```python
from build123d import *

# Parameters (mm, degrees)
F0_W      = 15.2
F0_H      = 19.2
F1_DEPTH  = 1.6
F2_R      = 1
F3_DEPTH  = 25
F4_W      = 10
F4_H      = 2.5
F5_DEPTH  = 2.5
F7_W      = 0.6
F7_H      = 0.6
F8_DEPTH  = 7.3
F9_W      = 0.6
F9_H      = 0.6
F10_DEPTH = 7.5
F11_R     = 3.473111
F12_DEPTH = 1
F13_R     = 2.5
F14_DEPTH = 7.5
F15_R     = 2.5


with BuildPart() as f1:
    # F0 (on Top) → F1 (new body)
    with BuildSketch(Plane.XY):
        Rectangle(F0_W, F0_H)
    extrude(amount=F1_DEPTH)

    # F2 (on face) → F3 (cut)
    with BuildSketch(Plane.XY.offset(1.6)):
        with Locations((-5.1, 7.1)):
            Circle(F2_R)
        with Locations((5.1, 7.1)):
            Circle(F2_R)
    extrude(amount=-F3_DEPTH, mode=Mode.SUBTRACT)

    # F4 (on face) → F5 (join)
    with BuildSketch(Plane.XY.offset(1.6)):
        with Locations((0, -7.85)):
            Rectangle(F4_W, F4_H)
    extrude(amount=F5_DEPTH)

    # F7 (on offset) → F8 (join)
    with BuildSketch(Plane.XY.offset(-1.5)):
        with Locations((3.85, -7.85)):
            Rectangle(F7_W, F7_H)
        with Locations((-3.85, -7.85)):
            Rectangle(F7_W, F7_H)
        with Locations((-1.35, -7.85)):
            Rectangle(F7_W, F7_H)
        with Locations((1.35, -7.85)):
            Rectangle(F7_W, F7_H)
        with Locations((1.35, -1.45)):
            Rectangle(F7_W, F7_H)
        with Locations((-1.35, -1.45)):
            Rectangle(F7_W, F7_H)
        with Locations((0, 1.45)):
            Rectangle(F7_W, F7_H)
        with Locations((-2.7, 1.45)):
            Rectangle(F7_W, F7_H)
    extrude(amount=F8_DEPTH)

    # F9 (on face) → F10 (join)
    with BuildSketch(Plane(origin=(0, -7.55, 0), x_dir=(-1, 0, 0), z_dir=(0, 1, 0))):
        with Locations((3.85, 5.5)):
            Rectangle(F9_W, F9_H)
        with Locations((-3.85, 5.5)):
            Rectangle(F9_W, F9_H)
        with Locations((1.35, 5.5)):
            Rectangle(F9_W, F9_H)
        with Locations((-1.35, 5.5)):
            Rectangle(F9_W, F9_H)
    extrude(amount=-F10_DEPTH)

    # F11 (on face) → F12 (join)
    with BuildSketch(Plane.XY.offset(5.8)):
        Circle(F11_R)
    extrude(amount=F12_DEPTH)

    # F13 (on face) → F14 (join)
    with BuildSketch(Plane.XY.offset(6.8)):
        Circle(F13_R)
    extrude(amount=F14_DEPTH)

    # F15
    f15_edges = [f1.edges().sort_by_distance(p)[0] for p in [
        (-2.5, 0, 14.3),
    ]]
    fillet(f15_edges, radius=F15_R)


solid = f1.part
```
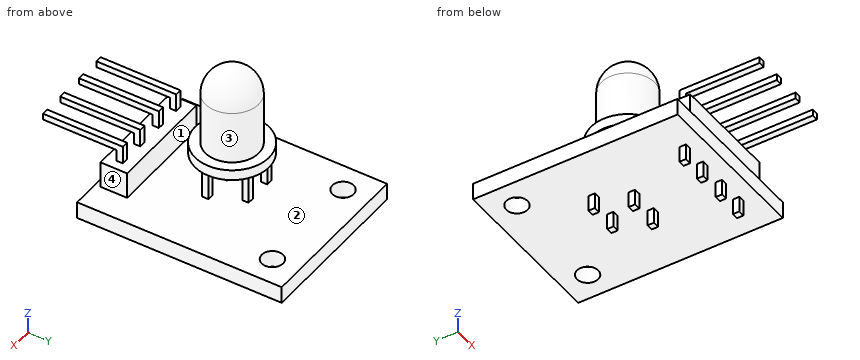
Geometry: final body of the model. Coordinates: model frame, mm. Face numbers are marked on the shaded views. A direction names the side the tool comes from. Round coordinates to 2 decimals unless told otherwise and drop trailing zeros. Write each loop counter-clockwise with the first axis right and the second up, starting at its lowest first coordinate (ties: lowest second). Pieces come first, ordered by that corner, then holes. Notation, with made-up numbers: M 48.5,86.5 L 65.5,86.5 A23 cw 65.5,107.5 Z; hole C -5.75,-12.5 d10. An arc over 180 degrees is marked long. Answer in a Markdown table with one row per item. Add a question column.
(1) Cut plane A-A, the plane y = 7.1. Return the cut outline in (x, z).
(2) Contact query for flat-ended pins moving along their axis: pin 1 (1.9 mm diameter, centred on y = -13, z = 5, fed in from -X); pin 2 (6 mm diameter, centred on x = -3, y = -2, fed in from -Z); pin 3 (3 mm diameter, centred on x = -2, y = -8, fed in from +Z); pin 4 (0.5 mm diameter, centred on x = -3, z = -0.5, fed in from +Y). Output: stop coordinate, or through.
(3) Draft query along Z for the marked faces 1 and 2. Return one class per face: pulls with the +Z half, pulls with the -Z half, needs draft (parallel to the pull), parting line crosses it, or undercut.
(4) Ray query, L1, parallel to Y at x = -0.25, z = 3.25; L2, parallel to Y at x = -5.1, z = 0.9; L3, parallel to Z at x = 1.75, y = -2.25. Return the intervals inside material, ascending.
(5) Cut plane D-D, the plane z = 5.5. Give the number of separate pieces and of enclosed holes in the cut face, then the cut area to 3 significant figures.
(6) Cut plane B-B, the plane y = 0. Return the cut outline in (x, z).
(7) Cut plane C-C, the plane x = 0. Return the cut outline in (y, z).
(8) Reachability of the marked faces 3 and 4 from +Z, -Z, +X, -X, +Y, -Y: full face, straight path, thin tool, end or side. Return the list, or none.
Established:
| question | item | result |
|---|---|---|
| 1 | outline | M -7.6,0 L -6.1,0 L -6.1,1.6 L -7.6,1.6 Z; M -4.1,0 L 4.1,0 L 4.1,1.6 L -4.1,1.6 Z; M 6.1,0 L 7.6,0 L 7.6,1.6 L 6.1,1.6 Z |
| 2 | pin 1 | x = -4.15 |
| 2 | pin 2 | z = -1.5 |
| 2 | pin 3 | z = 5.8 |
| 2 | pin 4 | y = 1.75 |
| 3 | face 1 | needs draft |
| 3 | face 2 | undercut |
| 4 | L1 | -9.1 to -6.6, 1.15 to 1.75 |
| 4 | L2 | -9.6 to 6.1, 8.1 to 9.6 |
| 4 | L3 | 0 to 1.6, 5.8 to 6.8 |
| 5 | separate pieces | 8 |
| 5 | enclosed holes | 0 |
| 5 | area | 19.4 mm² |
| 6 | outline | M -7.6,0 L 7.6,0 L 7.6,1.6 L -7.6,1.6 Z; M -3.47,5.8 L 3.47,5.8 L 3.47,6.8 L 2.5,6.8 L 2.5,11.8 A2.5 ccw -2.5,11.8 L -2.5,6.8 L -3.47,6.8 Z |
| 7 | outline | M -9.6,0 L 1.15,0 L 1.15,-1.5 L 1.75,-1.5 L 1.75,0 L 9.6,0 L 9.6,1.6 L 1.75,1.6 L 1.75,5.8 L 3.47,5.8 L 3.47,6.8 L 2.5,6.8 L 2.5,11.8 A2.5 ccw -2.5,11.8 L -2.5,6.8 L -3.47,6.8 L -3.47,5.8 L 1.15,5.8 L 1.15,1.6 L -6.6,1.6 L -6.6,4.1 L -9.1,4.1 L -9.1,1.6 L -9.6,1.6 Z |
| 8 | face 3 | +Z |
| 8 | face 4 | +Z, +X, +Y, -Y |
